Study the drawing (mm; zero at the part's minimum x, y, z) and answer. A direction names the side the tool comes from. Give positions to 0.01 mm unless a question says otherwise; leave off trailing zeros. Order: outer loops, then holes, each group sorted by start corner. A loop starts at its lowest first (then second) coordinate and runs counter-clockwise, first axis right, second up. Notation, with made-up numbers: (-28, 57.25) - (-2, 57.25) arc R34 ccw to (-2, 94.25) - close; hole circle Ø5 at (62, 71). An arc over 180 degrees is marked (long way). Put each result on its own line as item: value.
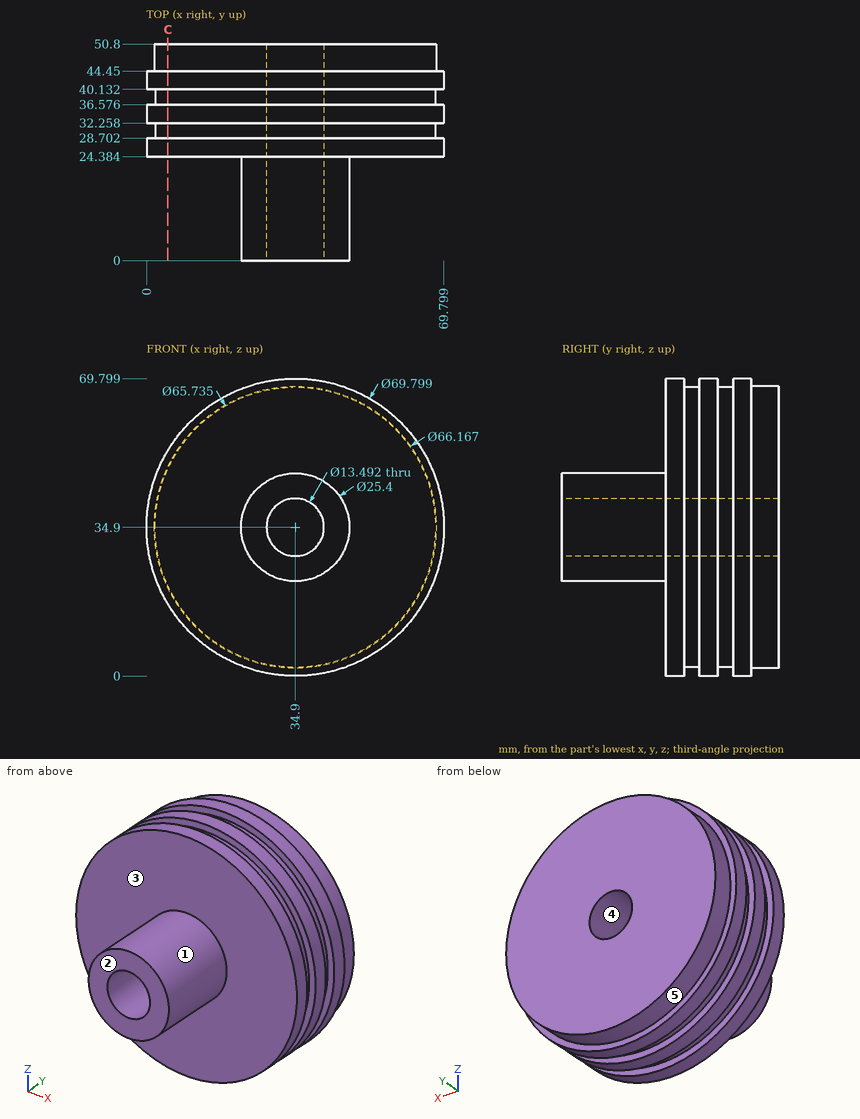
(1) A tool of negligible diameter and unlimited length cuts with its end or side. For the marked faces 1 and 2, from which of +Z, -Z, +X, -X, +Y, -Y can it reach the whole face along a straight path? Write none if from no direction.
Geometry check:
face 1: -Y
face 2: +Z, -Z, +X, -X, -Y
(2) Section C-C, the plane x = 5 is taken. Write down the section's boundary in (y, z).
Geometry check:
outline: (24.38, 16.9) - (28.7, 16.9) - (28.7, 21.25) - (32.26, 21.25) - (32.26, 16.9) - (36.58, 16.9) - (36.58, 21.25) - (40.13, 21.25) - (40.13, 16.9) - (44.45, 16.9) - (44.45, 20.74) - (50.8, 20.74) - (50.8, 49.06) - (44.45, 49.06) - (44.45, 52.9) - (40.13, 52.9) - (40.13, 48.55) - (36.58, 48.55) - (36.58, 52.9) - (32.26, 52.9) - (32.26, 48.55) - (28.7, 48.55) - (28.7, 52.9) - (24.38, 52.9) - close
(3) Given pin 1 (11 mm diameter, centred on x = 34.9, z = 34.9, fed in from -Y) (3 decimals); pin 2 (6 mm diameter, centred on y = 27.5, z = 16.5, fed in from -X); pin 3 (3 mm diameter, centred on x = 10, z = 20.5, fed in from -Y); pin 4 (1.5 mm diameter, centred on y = 32.5, z = 52.5, fed in from +X), each flat-ended and moving along its own axis, determine where each tip first touches the part or whether it passes through.
Geometry check:
pin 1: passes through
pin 2: stops at x = 3.58
pin 3: stops at y = 24.38
pin 4: stops at x = 65.46
(4) Determine the mould class of the marked faces 3, 4 and 5 for opening direction X: pulls with the +X half, pulls with the -X half, needs draft (parallel to the pull), parting line crosses it, or undercut.
Geometry check:
face 3: needs draft
face 4: undercut
face 5: parting line crosses it
(5) Straight lines are drawn through the part: line 1 (Y direction, x = 14, z = 62); line 2 (Y direction, x = 22, z = 6.5); line 3 (Z direction, x = 31, y = 6) (1 decimal). For each, find the intervals that lie inside material, in ascending order.
Geometry check:
line 1: y = 24.38 to 28.7, 32.26 to 36.58, 40.13 to 44.45
line 2: y = 24.38 to 50.8
line 3: z = 22.8 to 29.4, 40.4 to 47
